CAD build for the part. Positions are in the model's coordinates, mm. A direction names the side the tool comes from. Coordinates: 2 decimals unless noted, no trailing zeros. Order: outer loops, then holes, each group sorted by start corner. A loop starts at its lowest first (then second) coordinate and runs counter-clockwise, first axis right, second up.
from build123d import *

# Parameters (mm, degrees)
SKIZZE1_W                       = 60.8
SKIZZE1_H                       = 93.64
AUFSATZ_LINEAR_AUSTRAGEN1_DEPTH = 6
VERRUNDUNG1_R                   = 6
WANDUNG1_T                      = -1
SKIZZE2_W                       = 21.5
SKIZZE2_H                       = 9.5
SCHNITT_LINEAR_AUSTRAGEN1_DEPTH = 6
SKIZZE3_W                       = 22
SKIZZE3_H                       = 5
SCHNITT_LINEAR_AUSTRAGEN2_DEPTH = 6
SKIZZE4_W                       = 81.255814336
SKIZZE4_H                       = 48.084928105
SCHNITT_LINEAR_AUSTRAGEN3_DEPTH = 6


with BuildPart() as part:
    # Skizze1 → Aufsatz-Linear austragen1 (new body)
    with BuildSketch(Plane(origin=(0, 0, 0), x_dir=(0, 1, 0), z_dir=(0, 0, 1))):
        Rectangle(SKIZZE1_W, SKIZZE1_H)
    extrude(amount=AUFSATZ_LINEAR_AUSTRAGEN1_DEPTH)

    # Verrundung1
    verrundung1_edges = [part.edges().sort_by_distance(p)[0] for p in [
        (46.82, 30.4, 3),
        (46.82, -30.4, 3),
        (-46.82, -30.4, 3),
        (-46.82, 30.4, 3),
    ]]
    fillet(verrundung1_edges, radius=VERRUNDUNG1_R)

    # Wandung1
    wandung1_openings = [part.faces().sort_by_distance(p)[0] for p in [
        (0, 0, 6),
    ]]
    offset(amount=WANDUNG1_T, openings=wandung1_openings, kind=Kind.INTERSECTION)

    # Skizze2 → Schnitt-Linear austragen1 (cut)
    with BuildSketch(Plane.YZ.offset(46.82)):
        with Locations((0, 6)):
            Rectangle(SKIZZE2_W, SKIZZE2_H)
    extrude(amount=-SCHNITT_LINEAR_AUSTRAGEN1_DEPTH, mode=Mode.SUBTRACT)

    # Skizze3 → Schnitt-Linear austragen2 (cut)
    with BuildSketch(Plane.XZ.offset(30.4)):
        with Locations((-11.18, 3.5)):
            Rectangle(SKIZZE3_W, SKIZZE3_H)
    extrude(amount=-SCHNITT_LINEAR_AUSTRAGEN2_DEPTH, mode=Mode.SUBTRACT)

    # Skizze4 → Schnitt-Linear austragen3 (cut)
    with BuildSketch(Plane(origin=(0, 0, 0), x_dir=(1, 0, 0), z_dir=(0, 0, -1))):
        with Locations((0.624387115, -0.234506354)):
            Rectangle(SKIZZE4_W, SKIZZE4_H)
    extrude(amount=-SCHNITT_LINEAR_AUSTRAGEN3_DEPTH, mode=Mode.SUBTRACT)


solid = part.part
1) Slice it at C-C (z = 4.8). List the corners of the cut face in (x, y).
2) Which spindle directions (+Z, -Z, +X, -X, +Y, -Y) get a long thin tool onto all of the face, cutting with end or side? Do faces 4 (the cylindrical face through (-44.32, -27.97, 3.54)), 5 (the flat face through (46.82, 0, 1)). Say none if no direction does.
3) Slice it at D-D (x = 18). List the corners of the cut face in (y, z).
4) Slice it at B-B (y = -7). List the corners of the cut face in (x, z).
5) Drill centre lines: probe 1 along X at (y, z) = (22, 1.4); probe 2 along Y at (x, z) = (-35.5, 1.75); probe 3 along Z at (x, y) = (41.5, 0). Where is each one in solid material? Low to high.
6) Pin check, flat tips, straight feed: P1, Ø1.5, axis at y = 5.5, z = 3, coming from the +X side; P2, Ø1.1, axis at y = -30, z = 3, coming from the -X side; P3, Ø0.5, axis at x = 46.5, z = 5, coming from the -Y side. Stop position of each tip, or through.
7) Two-plate mould, pull along X, no slides. Class faces 1 (the flat face through (0, 25, 0)), 2 (the cylindrical face through (45.109, 28.596, 3.042)), 3 (the flat face through (-31, -29.4, 3)): released by +X, released by -X, zero draft, split by the parting line, or undercut.
8) Slice it at A-A (x = -4.5). List the corners of the cut face in (y, z).
Worked out:
1. outline: (-46.82, -24.4) arc R6 ccw to (-40.82, -30.4) - (-22.18, -30.4) - (-22.18, -29.4) - (-40.82, -29.4) arc R5 cw to (-45.82, -24.4) - (-45.82, 24.4) arc R5 cw to (-40.82, 29.4) - (40.82, 29.4) arc R5 cw to (45.82, 24.4) - (45.82, 10.75) - (46.82, 10.75) - (46.82, 24.4) arc R6 ccw to (40.82, 30.4) - (-40.82, 30.4) arc R6 ccw to (-46.82, 24.4) - close; (-0.18, -30.4) - (40.82, -30.4) arc R6 ccw to (46.82, -24.4) - (46.82, -10.75) - (45.82, -10.75) - (45.82, -24.4) arc R5 cw to (40.82, -29.4) - (-0.18, -29.4) - close
2. face 4: +Z
2. face 5: +Z, -Z, +X, +Y, -Y
3. outline: (-30.4, 0) - (-23.81, 0) - (-23.81, 1) - (-29.4, 1) - (-29.4, 6) - (-30.4, 6) - close; (24.28, 0) - (30.4, 0) - (30.4, 6) - (29.4, 6) - (29.4, 1) - (24.28, 1) - close
4. outline: (-46.82, 0) - (-40, 0) - (-40, 1) - (-45.82, 1) - (-45.82, 6) - (-46.82, 6) - close; (41.25, 0) - (46.82, 0) - (46.82, 1.25) - (45.82, 1.25) - (45.82, 1) - (41.25, 1) - close
5. probe 1: x = -46.82 to -45.82, 45.82 to 46.82
5. probe 2: y = -30.4 to -29.4, 29.4 to 30.4
5. probe 3: z = 0 to 1
6. P1: stops at x = -45.82
6. P2: stops at x = -44.06
6. P3: stops at y = -26.95
7. face 1: zero draft
7. face 2: released by +X
7. face 3: undercut
8. outline: (-30.4, 0) - (-23.81, 0) - (-23.81, 1) - (-30.4, 1) - close; (24.28, 0) - (30.4, 0) - (30.4, 6) - (29.4, 6) - (29.4, 1) - (24.28, 1) - close
